Build history of the part. All positions in model axes, mm. Round coordinates to 2 decimals unless told otherwise and drop trailing zeros. Order: outer loops, then holes, each group sorted by start corner. A loop starts at its lowest first (then second) coordinate and runs counter-clockwise, first axis right, second up. Notation, with made-up numbers: (-13, 66) -> (31, 66) arc R31 cw to (31, 102) -> close; hole circle Ø4 at (54, 47). An arc over 180 degrees is marked (long way). Write item = value, one per line.
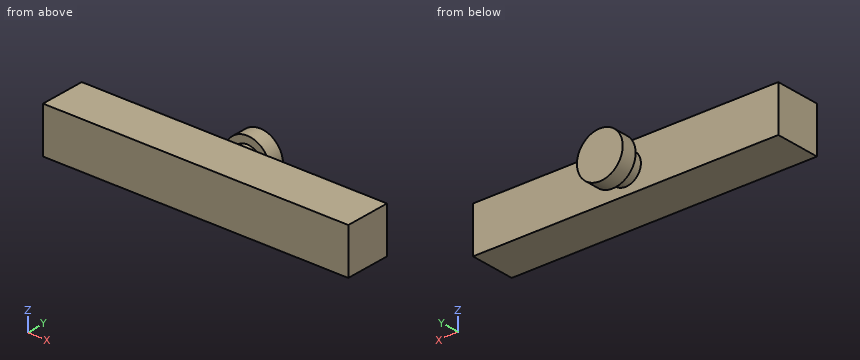
from build123d import *

# Parameters (mm, degrees)
SKETCH1_W           = 200
SKETCH1_H           = 60
BOSS_EXTRUDE1_DEPTH = 30
SKETCH2_R           = 10
BOSS_EXTRUDE3_DEPTH = 10
SKETCH3_R           = 15
BOSS_EXTRUDE4_DEPTH = 10
SKETCH4_W           = 200
SKETCH4_H           = 15
CUT_EXTRUDE1_DEPTH  = 50


with BuildPart() as part:
    # Sketch1 → Boss-Extrude1 (new body)
    with BuildSketch(Plane(origin=(0, 0, 0), x_dir=(1, 0, 0), z_dir=(0, 1, 0))):
        with Locations((100, -30)):
            Rectangle(SKETCH1_W, SKETCH1_H)
    extrude(amount=-BOSS_EXTRUDE1_DEPTH)

    # Sketch2 → Boss-Extrude3 (add)
    with BuildSketch(Plane(origin=(0, 0, 0), x_dir=(1, 0, 0), z_dir=(0, 1, 0))):
        with Locations(Location((100, -30, 0), (0, 0, 90))):
            Circle(SKETCH2_R)
    extrude(amount=BOSS_EXTRUDE3_DEPTH)

    # Sketch3 → Boss-Extrude4 (add)
    with BuildSketch(Plane(origin=(0, 10, 0), x_dir=(1, 0, 0), z_dir=(0, 1, 0))):
        with Locations(Location((100, -30, 0), (0, 0, 270))):
            Circle(SKETCH3_R)
    extrude(amount=BOSS_EXTRUDE4_DEPTH)

    # Sketch4 → Cut-Extrude1 (cut)
    with BuildSketch(Plane(origin=(0, 0, 0), x_dir=(1, 0, 0), z_dir=(0, 1, 0))):
        with Locations((100, -7.5)):
            Rectangle(SKETCH4_W, SKETCH4_H)
        with Locations((100, -52.5)):
            Rectangle(SKETCH4_W, SKETCH4_H)
    extrude(amount=-CUT_EXTRUDE1_DEPTH, mode=Mode.SUBTRACT)


solid = part.part
Q1. Flat gauge pin, fed straight in: pin 1 (1 mm diameter, centred on y = -21.5, z = 19.5, fed in from -X). Where does the tip first touch, or does it go through?
Check values:
pin_1 = 0
Q2. Cut at A-A, the plane x = 100. List the corners of the cut face in (y, z), and give its area (3 significant figures).
Check values:
outline = (-30, 15) -> (0, 15) -> (0, 20) -> (10, 20) -> (10, 15) -> (20, 15) -> (20, 45) -> (10, 45) -> (10, 40) -> (0, 40) -> (0, 45) -> (-30, 45) -> close
area = 1,400 mm²
Q3. Probe probe 1 along Y at (x, z) = (111.5, 22.25); probe 2 along Y at (x, z) = (14, 26); probe 3 along X at (y, z) = (1, 35.75). List the from-to ranges inside material, lowest first.
Check values:
probe_1 = -30 to 0, 10 to 20
probe_2 = -30 to 0
probe_3 = 91.82 to 108.18
Q4. Cut at C-C, the plane x = 65. List the corners of the cut face in (y, z).
Check values:
outline = (-30, 15) -> (0, 15) -> (0, 45) -> (-30, 45) -> close
Q5. Cut at B-B, the plane z = 30. List the corners of the cut face in (x, y).
Check values:
outline = (0, -30) -> (200, -30) -> (200, 0) -> (110, 0) -> (110, 10) -> (115, 10) -> (115, 20) -> (85, 20) -> (85, 10) -> (90, 10) -> (90, 0) -> (0, 0) -> close
